Design review of the part built by this model. Coordinates are the model's own, in mm. A direction names the side the tool comes from. Round coordinates to 2 decimals unless told otherwise and drop trailing zeros. Write each loop counter-clockwise with the first axis right and the second up, starting at its lowest first coordinate (ties: lowest second). Pieces come first, ordered by that corner, then holes. Notation, with made-up numbers: (62.5, 53.25) - (114.5, 53.25) arc R13 cw to (114.5, 77.25) - close; hole circle Ø1 at (35, 74). An arc over 180 degrees is marked (long way). Use one line per item in the form item = value.
```python
from build123d import *

# Parameters (mm, degrees)
SKETCH1_W           = 152.4
SKETCH1_H           = 76.2
BOSS_EXTRUDE1_DEPTH = 1219.2
FILLET1_R           = 17.78
CHAMFER1_SIZE       = 25.4
SKETCH2_W           = 1290.477589614
SKETCH2_H           = 141.513172698
SKETCH2_W_2         = 738.880843562
SKETCH2_H_2         = 106.185211378
BOSS_EXTRUDE2_DEPTH = 25.4
SKETCH3_W           = 145.88030373
SKETCH3_H           = 116.073932347
BOSS_EXTRUDE3_DEPTH = 152.4
SKETCH4_W           = 11.32867816
SKETCH4_H           = 11.32867816
BOSS_EXTRUDE4_DEPTH = 101.6
SKETCH5_W           = 41.535496856
SKETCH5_H           = 41.006382246
BOSS_EXTRUDE5_DEPTH = 53.34
SKETCH6_R           = 56.660477504
BOSS_EXTRUDE6_DEPTH = 53.34
SKETCH7_R           = 47.532369055
SKETCH7_R_2         = 57.711896929
BOSS_EXTRUDE7_DEPTH = 53.34
SKETCH8_W           = 11.310933435
SKETCH8_H           = 106.185211378
BOSS_EXTRUDE8_DEPTH = 76.2


with BuildPart() as part:
    # Sketch1 → Boss-Extrude1 (new body)
    with BuildSketch(Plane.XY):
        Rectangle(SKETCH1_W, SKETCH1_H)
    extrude(amount=BOSS_EXTRUDE1_DEPTH)

    # Fillet1
    fillet1_edges = [part.edges().sort_by_distance(p)[0] for p in [
        (0, 38.1, 0),
    ]]
    fillet(fillet1_edges, radius=FILLET1_R)

    # Chamfer1
    chamfer1_edges = [part.edges().sort_by_distance(p)[0] for p in [
        (0, -38.1, 1219.2),
    ]]
    chamfer(chamfer1_edges, length=CHAMFER1_SIZE)

    # Sketch2 → Boss-Extrude2 (add)
    with BuildSketch(Plane(origin=(0, 38.1, 0), x_dir=(1, 0, 0), z_dir=(0, 1, 0))):
        with Locations((0, -507.012478725)):
            Rectangle(SKETCH2_W, SKETCH2_H)
        with Locations((0, -1162.865725204)):
            Rectangle(SKETCH2_W_2, SKETCH2_H_2)
    extrude(amount=BOSS_EXTRUDE2_DEPTH)

    # Sketch3 → Boss-Extrude3 (add)
    with BuildSketch(Plane(origin=(0, 63.5, 0), x_dir=(1, 0, 0), z_dir=(0, 1, 0))):
        with Locations((0, -507.950753796)):
            Rectangle(SKETCH3_W, SKETCH3_H)
    extrude(amount=BOSS_EXTRUDE3_DEPTH)

    # Sketch4 → Boss-Extrude4 (add)
    with BuildSketch(Plane.ZY.offset(72.940151865)):
        with Locations((507.221293342, 169.657361137)):
            Rectangle(SKETCH4_W, SKETCH4_H)
    boss_extrude4 = extrude(amount=BOSS_EXTRUDE4_DEPTH)

    # Sketch5 → Boss-Extrude5 (add)
    with BuildSketch(Plane.ZY.offset(174.540151865)):
        with Locations((505.573109598, 171.765287406)):
            Rectangle(SKETCH5_W, SKETCH5_H)
    boss_extrude5 = extrude(amount=BOSS_EXTRUDE5_DEPTH)

    # Sketch6 → Boss-Extrude6 (add)
    with BuildSketch(Plane(origin=(0, 0, 484.80536117), x_dir=(-1, 0, 0), z_dir=(0, 0, -1))):
        with Locations((201.337814598, 173.008334857)):
            Circle(SKETCH6_R)
    boss_extrude6 = extrude(amount=BOSS_EXTRUDE6_DEPTH)

    # Mirror1: Boss-Extrude4, Boss-Extrude5, Boss-Extrude6 across plane
    add(boss_extrude4.mirror(Plane(origin=(0, 0, 0), x_dir=(0, 0, 1), z_dir=(1, 0, 0))))
    add(boss_extrude5.mirror(Plane(origin=(0, 0, 0), x_dir=(0, 0, 1), z_dir=(1, 0, 0))))
    add(boss_extrude6.mirror(Plane(origin=(0, 0, 0), x_dir=(0, 0, 1), z_dir=(1, 0, 0))))

    # Sketch7 → Boss-Extrude7 (add)
    with BuildSketch(Plane(origin=(0, 38.1, 0), x_dir=(1, 0, 0), z_dir=(0, 1, 0))):
        with Locations((0, -64.420131153)):
            Circle(SKETCH7_R)
        with Locations((0, -1030.4765592)):
            Circle(SKETCH7_R_2)
    extrude(amount=BOSS_EXTRUDE7_DEPTH)

    # Sketch8 → Boss-Extrude8 (add)
    with BuildSketch(Plane(origin=(0, 63.5, 0), x_dir=(1, 0, 0), z_dir=(0, 1, 0))):
        with Locations((363.784955063, -1162.865725204)):
            Rectangle(SKETCH8_W, SKETCH8_H)
    boss_extrude8 = extrude(amount=BOSS_EXTRUDE8_DEPTH)

    # Mirror2: Boss-Extrude8 across plane
    add(boss_extrude8.mirror(Plane(origin=(0, 0, 0), x_dir=(0, 0, 1), z_dir=(1, 0, 0))))


solid = part.part
```
Q1. We need section D-D on x = -536.5. Write out the cut boundary in (y, z), then the cut area to 3 significant figures.
Calculated:
outline = (38.1, 436.26) - (63.5, 436.26) - (63.5, 577.77) - (38.1, 577.77) - close
area = 3,590 mm2
Q2. We need section B-B on x = 105.5. Write out the cut boundary in (y, z).
Calculated:
outline = (38.1, 436.26) - (63.5, 436.26) - (63.5, 577.77) - (38.1, 577.77) - close; (38.1, 1109.77) - (63.5, 1109.77) - (63.5, 1215.96) - (38.1, 1215.96) - close; (163.99, 501.56) - (175.32, 501.56) - (175.32, 512.89) - (163.99, 512.89) - close
Q3. Machinability: for faces 4 (the flat face through (221, 38.1, 1162)), 5 (the flat face through (-201, 171, 526.341)), 6 (the flat face through (2, 47, 1109.773)), 7 (the flat face through (201, 151.262, 505)), 8 (the flat face through (358.129, 101, 1164)), which of the approach directions +Z, -Z, +X, -X, +Y, -Y give a long, thin tool a straight path to every point of the face, cutting with its end or side? Answer none if there is none.
Calculated:
face_4 = +Z, -Z, +X, -Y
face_5 = +Z, -X, +Y
face_6 = +X, -X, +Y
face_7 = +Z, +X
face_8 = +Z, -Z, +Y
Q4. To check wall thickness, follow line 1 along Y through (x, z) = (338.5, 440.5); line 2 along X through (y, z) = (29, 808.5); line 3 along Z through (x, y) = (51, 72). State the ranges of each line that lie inside material, in increasing order. Write a range as from..to.
Calculated:
line_1 = 38.1..63.5
line_2 = -76.2..76.2
line_3 = 449.91..565.99, 1003.46..1057.49
Q5. We need section A-A on x = -276.5. Write out the cut boundary in (y, z).
Calculated:
outline = (38.1, 436.26) - (63.5, 436.26) - (63.5, 577.77) - (38.1, 577.77) - close; (38.1, 1109.77) - (63.5, 1109.77) - (63.5, 1215.96) - (38.1, 1215.96) - close
Q6. We need section C-C on z = 185. Write out the cut boundary in (x, y), then the cut area to 3 significant figures.
Calculated:
outline = (-76.2, -38.1) - (76.2, -38.1) - (76.2, 38.1) - (-76.2, 38.1) - close
area = 11,600 mm2
Q7. Draft analysis for pull direction Y (two halves, no side actions). For faces 1 (the flat face through (-201, 149, 484.805)), 2 (the flat face through (-1, -8, 0)), 3 (the flat face through (-365, 38.1, 506)), state which applies: released by +Y, released by -Y, zero draft, split by the parting line, or undercut.
Calculated:
face_1 = undercut
face_2 = zero draft
face_3 = released by -Y
Q8. For P1, Ø10, axis at y = 161.5, z = 436, coming from the -X side; P2, Ø23, axis at y = 10.5, z = 693, coming from the -X side; P3, Ø12.5, axis at y = 172, z = 510.5, coming from the +X side, all flat-tipped, find the tip position at first contact; note any pin that passes through.
Calculated:
P1 = -257.62
P2 = -76.2
P3 = 227.88
